```python
from build123d import *

# Parameters (mm, degrees)
SKETCH1_W           = 47
SKETCH1_H           = 25
BOSS_EXTRUDE1_DEPTH = 10
SKETCH2_R           = 2
CUT_EXTRUDE1_DEPTH  = 8
SKETCH5_W           = 30
SKETCH5_H           = 18
CUT_EXTRUDE2_DEPTH  = 10


with BuildPart() as part:
    # Sketch1 → Boss-Extrude1 (new body)
    with BuildSketch(Plane(origin=(0, 0, 0), x_dir=(1, 0, 0), z_dir=(0, 1, 0))):
        with Locations((23.5, 12.5)):
            Rectangle(SKETCH1_W, SKETCH1_H)
    extrude(amount=BOSS_EXTRUDE1_DEPTH)

    # Sketch2 → Cut-Extrude1 (cut)
    with BuildSketch(Plane(origin=(0, 10, 0), x_dir=(1, 0, 0), z_dir=(0, 1, 0))):
        with Locations((3, 12.5)):
            Circle(SKETCH2_R)
        with Locations((44, 12.5)):
            Circle(SKETCH2_R)
    extrude(amount=-CUT_EXTRUDE1_DEPTH, mode=Mode.SUBTRACT)

    # Sketch5 → Cut-Extrude2 (cut)
    with BuildSketch(Plane(origin=(0, 10, 0), x_dir=(1, 0, 0), z_dir=(0, 1, 0))):
        with Locations((23.5, 12.5)):
            Rectangle(SKETCH5_W, SKETCH5_H)
    extrude(amount=-CUT_EXTRUDE2_DEPTH, mode=Mode.SUBTRACT)


solid = part.part
```
Part model, mm, in its own coordinate system. A direction names the side the tool comes from. Give positions to 0.01 mm unless a question says otherwise; leave off trailing zeros. Write each loop counter-clockwise with the first axis right and the second up, starting at its lowest first coordinate (ties: lowest second). Pieces come first, ordered by that corner, then holes. Notation, with made-up numbers: (34, -4.5) -> (65, -4.5) arc R7 cw to (65, 1.5) -> close; hole circle Ø3 at (61.5, 45). An arc over 180 degrees is marked (long way). Put each result on its own line as item: value. Start each with the question number.
Item 1: Pull direction Z, two halves, no side cores. Call faces 4 (the face through (23, 5, -25)), 5 (the face through (23, 5, -3.5)), 6 (the face through (23, 5, 0)), 7 (the face through (23, 10, -2)): pulls with the +Z half, pulls with the -Z half, needs draft (parallel to the pull), parting line crosses it, or undercut.
Item 2: Cut at D-D (y = 5). List the corners of the cut face in (x, z), then the cut area to 3 significant figures.
Item 3: Wall check: L1, parallel to X at y = 4, z = -12.5; L2, parallel to X at y = 3.75, z = -5.5; L3, parallel to Z at x = 37, y = 4. Give the ranges that are in metal, low to high. Write a range as [from, to].
Item 4: Cut at A-A (z = -12.5). List the corners of the cut face in (x, y), then the cut area to 3 significant figures.
Item 5: Cut at C-C (x = 13). List the corners of the cut face in (y, z).
Item 6: Pin check, flat tips, straight feed: pin 1 Ø2 at (x, z) = (37, -17) entering from -Y; pin 2 Ø3 at (x, z) = (3, -12.5) entering from +Y. Stop position of each tip, or through.
Item 7: Cut at B-B (x = 3). List the corners of the cut face in (y, z).
Item 8: Which spindle directions (+Z, -Z, +X, -X, +Y, -Y) get a long thin tool onto all of the face, cutting with end or side? Do faces 1 (the face through (23, 0, -2)), 2 (the face through (38.5, 5, -12)), 3 (the face through (44, 2, -13)). Say none if no direction does.
Answer list:
1. face 4: pulls with the -Z half
1. face 5: undercut
1. face 6: pulls with the +Z half
1. face 7: needs draft
2. outline: (0, -25) -> (47, -25) -> (47, 0) -> (0, 0) -> close; hole circle Ø4 at (3, -12.5); hole (8.5, -21.5) -> (38.5, -21.5) -> (38.5, -3.5) -> (8.5, -3.5) -> close; hole circle Ø4 at (44, -12.5)
2. area: 610 mm2
3. L1: x = [0, 1], [5, 8.5], [38.5, 42], [46, 47]
3. L2: x = [0, 8.5], [38.5, 47]
3. L3: z = [-25, -21.5], [-3.5, 0]
4. outline: (0, 0) -> (8.5, 0) -> (8.5, 10) -> (5, 10) -> (5, 2) -> (1, 2) -> (1, 10) -> (0, 10) -> close; (38.5, 0) -> (47, 0) -> (47, 10) -> (46, 10) -> (46, 2) -> (42, 2) -> (42, 10) -> (38.5, 10) -> close
4. area: 106 mm2
5. outline: (0, -25) -> (10, -25) -> (10, -21.5) -> (0, -21.5) -> close; (0, -3.5) -> (10, -3.5) -> (10, 0) -> (0, 0) -> close
6. pin 1: passes through
6. pin 2: stops at y = 2
7. outline: (0, -25) -> (10, -25) -> (10, -14.5) -> (2, -14.5) -> (2, -10.5) -> (10, -10.5) -> (10, 0) -> (0, 0) -> close
8. face 1: +Z, -Z, +X, -X, -Y
8. face 2: +Y, -Y
8. face 3: +Y
